from build123d import *

# Parameters (mm, degrees)
SKETCH_1_R      = 4.6
EXTRUDE_1_DEPTH = 5
SKETCH_2_R      = 1.24
EXTRUDE_2_DEPTH = 3.5
FILLET_1_SIZE   = 1
FILLET_2_SIZE   = 1.2


with BuildPart() as part:
    # 草图1 → 凸台-拉伸1 (new body)
    with BuildSketch(Plane.XY):
        Circle(SKETCH_1_R)
    extrude(amount=EXTRUDE_1_DEPTH)

    # 草图2 → 凸台-拉伸2 (add)
    with BuildSketch(Plane.XY.offset(5)):
        Circle(SKETCH_2_R)
    extrude(amount=EXTRUDE_2_DEPTH)

    # 圆角1
    # a fillet whose section is not a circle: 1 mm, written as the material it takes off along each edge
    with BuildSketch(Plane(origin=(0, 0, 8.5), x_dir=(1, 0, 0), z_dir=(0, -1, 0))) as fillet_1_piece_1:
        with BuildLine():
            Bezier((1.24, -FILLET_1_SIZE), (1.24, 0), (1.24 - FILLET_1_SIZE, 0), weights=[1, 0.070710678, 1])
            Line((1.24 - FILLET_1_SIZE, 0), (1.24, 0))
            Line((1.24, 0), (1.24, -FILLET_1_SIZE))
        make_face()
    revolve(axis=Axis((0, 0, 8.5), (0, 0, 1)), mode=Mode.SUBTRACT)

    # 圆角2
    # a fillet whose section is not a circle: 1.2 mm, written as the material it takes off along each edge
    with BuildSketch(Plane(origin=(0, 0, 0), x_dir=(1, 0, 0), z_dir=(0, -1, 0))) as fillet_2_piece_1:
        with BuildLine():
            Bezier((4.6, FILLET_2_SIZE), (4.6, 0), (4.6 - FILLET_2_SIZE, 0), weights=[1, 0.084852814, 1])
            Line((4.6 - FILLET_2_SIZE, 0), (4.6, 0))
            Line((4.6, 0), (4.6, FILLET_2_SIZE))
        make_face()
    revolve(axis=Axis((0, 0, 0), (0, 0, 1)), mode=Mode.SUBTRACT)


solid = part.part
For this review, take the finished solid that the model builds, in its own axes (mm). A direction names the side the tool comes from. Coordinates: 2 decimals unless noted, no trailing zeros. Loops run counter-clockwise (first coordinate to the right, second up) from the corner with the lowest first, then second, coordinate; pieces in that order, holes last. Notation, with made-up numbers: (-12.5, 15) - (42.5, 15) arc R11 ccw to (42.5, 24) - close; hole circle Ø8 at (58, 2). An arc over 180 degrees is marked (long way). Return JSON: item names as keys, results as strings.
Item 1: For faces 1 (the cylindrical face through (-3.65, -2.8, 3.07)), 2 (the flat face through (1, -1, 5)), list the 3-axis set-ups (+Z, -Z, +X, -X, +Y, -Y) from which the entire face can be reached by the end or side of a thin tool; tool diameter is ignored.
Determined:
{"face 1": "+Z, -Z", "face 2": "+Z"}
Item 2: Insertion check: pin 1 (1.5 mm diameter, centred on x = -0.5, z = 6.5, fed in from +Y); pin 2 (4 mm diameter, centred on x = -3.5, y = -3, fed in from +Z); pin 3 (4 mm diameter, centred on y = -3, z = 3.5, fed in from -X). Each pin has a flat end and moves straight along its axis. Give the tip position at first contact, or say it passes through.
Determined:
{"pin 1": "stops at y = 1.24", "pin 2": "stops at z = 5", "pin 3": "stops at x = -4.49"}
Item 3: Take a section at A-A (z = 5.25). Give the boundary of the cut face in (x, y), then the cut area to 3 significant figures.
Determined:
{"outline": "circle Ø2.48 at (0, 0)", "area": "4.83 mm2"}
Item 4: Take a section at B-B (z = 2.5). Give the boundary of the cut face in (x, y).
Determined:
{"outline": "circle Ø9.2 at (0, 0)"}
Item 5: For line 1 (Z direction, x = -3, y = 0.5); line 2 (Z direction, x = 0, y = 0.75); line 3 (X direction, y = 1, z = 3.25), list the stretches that pass through material, from the lowest coordinate up.
Determined:
{"line 1": "z = 0 to 5", "line 2": "z = 0 to 8.06", "line 3": "x = -4.49 to 4.49"}
